Geometry check sheet. Reference: drawing and pictorial views, mm from the part's lowest x, y, z. A direction names the side the tool comes from. Coordinates: 2 decimals unless noted, no trailing zeros. Loops run counter-clockwise (first coordinate to the right, second up) from the corner with the lowest first, then second, coordinate; pieces in that order, holes last. Notation, with made-up numbers: (60.5, -29) -> (73.5, -29) arc R16 ccw to (73.5, -20) -> close; hole circle Ø2 at (57.25, -8.75). An arc over 180 degrees is marked (long way). Answer as a JSON object with one key per item and string values. Group by question number.
Q1. Cross-section at A-A on z = 5. Record the boundary of the cut face in (x, y).
Q2. Cross-section at C-C on z = 12. Record the boundary of the cut face in (x, y).
Q3. Set-up check for the marked faces 1 and 2: record each of +Z, -Z, +X, -X, +Y, -Y from which the full face is reachable in a straight line by a thin tool's end or side.
Q4. Scan lines: L1, parallel to Y at x = 5, z = 8.5; L2, parallel to Y at x = 8.75, z = 18; L3, parallel to Z at x = 13, y = 11.5. Record each from-to range of solid material in increasing order.
Q5. Cross-section at D-D on y = 43. Record the boundary of the cut face in (x, z), and give its area (3 significant figures).
Q6. Gauge pin test, flat ends, axial feed: pin 1 Ø0.6 at (x, y) = (6.5, 52.5) entering from +Z; pin 2 Ø6 at (x, y) = (13.5, 36) entering from +Z; pin 3 Ø5.5 at (x, z) = (7.5, 28.5) entering from -Y. Record the tip position at first contact, or that the pin passes through.
Q7. Cross-section at B-B on x = 10. Record the boundary of the cut face in (y, z), and give its area (3 significant figures).
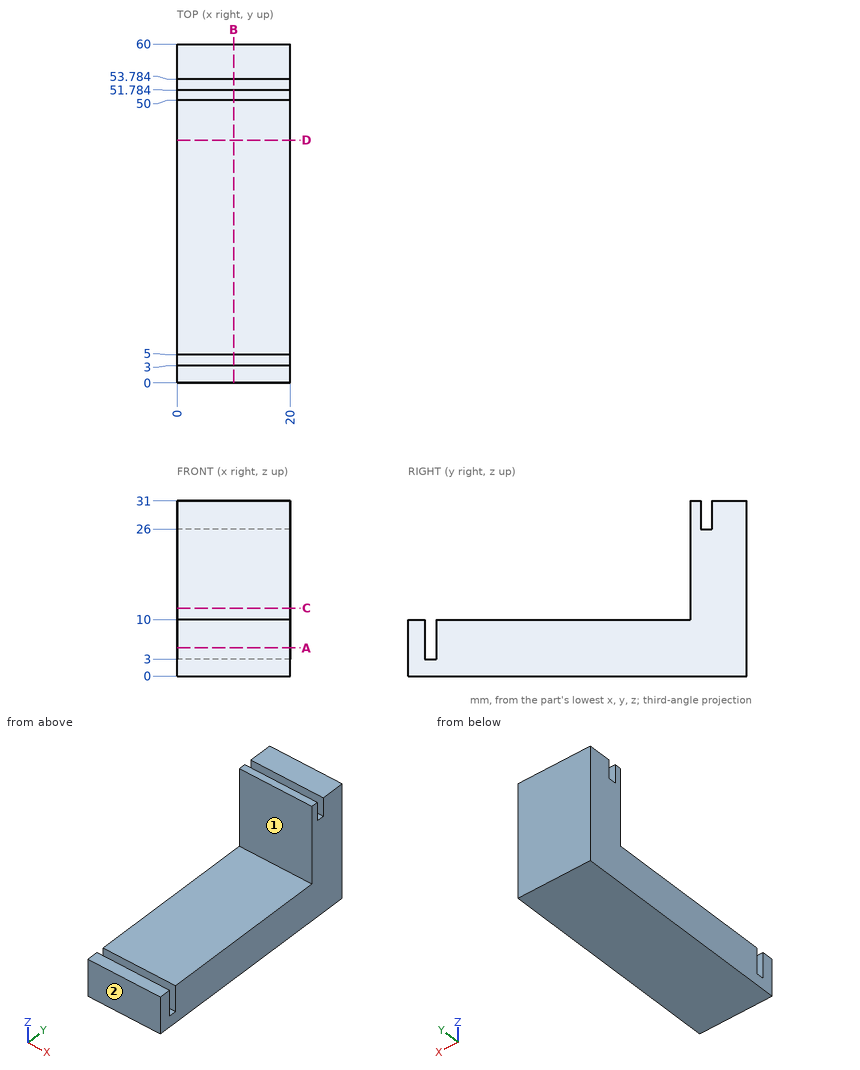
Computed values:
{
 "1": {"outline": "(0, 0) -> (20, 0) -> (20, 3) -> (0, 3) -> close; (0, 5) -> (20, 5) -> (20, 60) -> (0, 60) -> close"},
 "2": {"outline": "(0, 50) -> (20, 50) -> (20, 60) -> (0, 60) -> close"},
 "3": {"face 1": "+Z, +X, -X, -Y", "face 2": "+Z, -Z, +X, -X, -Y"},
 "4": {"L1": "y = 0 to 3, 5 to 60", "L2": "y = 50 to 60", "L3": "z = 0 to 10"},
 "5": {"outline": "(0, 0) -> (20, 0) -> (20, 10) -> (0, 10) -> close", "area": "200 mm²"},
 "6": {"pin 1": "stops at z = 26", "pin 2": "stops at z = 10", "pin 3": "stops at y = 50"},
 "7": {"outline": "(0, 0) -> (60, 0) -> (60, 31) -> (53.78, 31) -> (53.78, 26) -> (51.78, 26) -> (51.78, 31) -> (50, 31) -> (50, 10) -> (5, 10) -> (5, 3) -> (3, 3) -> (3, 10) -> (0, 10) -> close", "area": "786 mm²"}
}
